For this review, take the finished solid that the model builds, in its own axes (mm). A direction names the side the tool comes from. Coordinates: 2 decimals unless noted, no trailing zeros. Write each loop counter-clockwise with the first axis right and the second up, starting at its lowest first coordinate (ties: lowest second). Pieces come first, ordered by that corner, then holes. Notation, with made-up numbers: (-25, 36) - (33, 36) arc R25 cw to (33, 57) - close; hole circle Ø8 at (-14, 56). An arc over 180 degrees is marked (long way). Use one line per item in the form item = value. Start each with the question number.
1) We need section D-D (x = 29.5). Give the boundary of the cut face in (y, z).
2) We need section B-B (x = 135). Give the boundary of the cut face in (y, z) (3 decimals), plus the area to 3 significant figures.
3) Tool access review of faces 4 (the flat face through (152, 152, 9.525)), 5 (the flat face through (150, 361, 0)): name each direction out of +Z, -Z, +X, -X, +Y, -Y from which nothing blocks a thin tool from reaching the whole face with its end or side.
4) We need section A-A (z = 5). Give the boundary of the cut face in (x, y).
5) We need section C-C (y = 54.5). Give the boundary of the cut face in (x, z).
6) For L1, parallel to Y at x = 154, z = 1.5; L2, parallel to Y at x = 148.5, z = 4.25; L3, parallel to Y at x = 25, z = 1.5, list the stretches that pass through material, from the lowest coordinate up. Write a range as from..to.
7) Mouldability with a two-part tool opening along Y and no side actions: class faces 1 (the cylindrical face through (127.025, 151.283, 4.696)), 2 (the flat face through (155, 711.2, 9)), 3 (the flat face through (0, 436, 9)) as pulls with the +Y half, pulls with the -Y half, needs draft (parallel to the pull), parting line crosses it, or undercut.
```python
from build123d import *

# Parameters (mm, degrees)
F1_DEPTH = 19.05
F2_R     = 25.4
F3_DEPTH = 9.525


with BuildPart() as f1:
    # F0 (on Top) → F1 (new body)
    with BuildSketch(Plane.XY):
        with BuildLine():
            Line((0, 711.2), (0, 152.4))
            ThreePointArc((0, 152.4), (44.636927, 44.636927), (152.4, 0))
            ThreePointArc((152.4, 0), (260.163073, 44.636927), (304.8, 152.4))
            Line((304.8, 152.4), (304.8, 711.2))
            Line((304.8, 711.2), (0, 711.2))
        make_face()
    extrude(amount=F1_DEPTH)

    # F2 (on face) → F3 (cut)
    with BuildSketch(Plane(origin=(0, 0, 0), x_dir=(1, 0, 0), z_dir=(0, 0, -1))):
        with Locations((152.4, -152.4)):
            Circle(F2_R)
    extrude(amount=-F3_DEPTH, mode=Mode.SUBTRACT)


solid = f1.part
```
Determined:
q1.outline = (62.28, 0) - (711.2, 0) - (711.2, 19.05) - (62.28, 19.05) - close
q2.outline = (0.997, 0) - (133.896, 0) - (133.896, 9.525) - (170.904, 9.525) - (170.904, 0) - (711.2, 0) - (711.2, 19.05) - (0.997, 19.05) - close
q2.area = 13,200 mm²
q3.face_4 = -Z
q3.face_5 = -Z, +X, -X, +Y, -Y
q4.outline = (0, 152.4) arc R152.4 ccw to (152.4, 0) arc R152.4 ccw to (304.8, 152.4) - (304.8, 711.2) - (0, 711.2) - close; hole circle Ø50.8 at (152.4, 152.4)
q5.outline = (35.6, 0) - (269.2, 0) - (269.2, 19.05) - (35.6, 19.05) - close
q6.L1 = 0.01..127.05, 177.75..711.2
q6.L2 = 0.05..127.3, 177.5..711.2
q6.L3 = 68.76..711.2
q7.face_1 = undercut
q7.face_2 = pulls with the +Y half
q7.face_3 = needs draft
